The drawing under review shows one solid part. Ordinate dimensions are in mm from its lowest x, y, z. Coordinates: 2 decimals unless noted, no trailing zeros. Write each loop counter-clockwise with the first axis right and the second up, starting at its lowest first coordinate (ties: lowest second). Pieces come first, ordered by that corner, then holes. Notation, with made-up numbers: (-29, 16.25) - (7, 16.25) arc R16 cw to (7, 40.25) - close; hole circle Ø5 at (67, 27). An arc over 180 degrees is marked (long way). Answer as CSV lines item,"result". Start each with the question number.
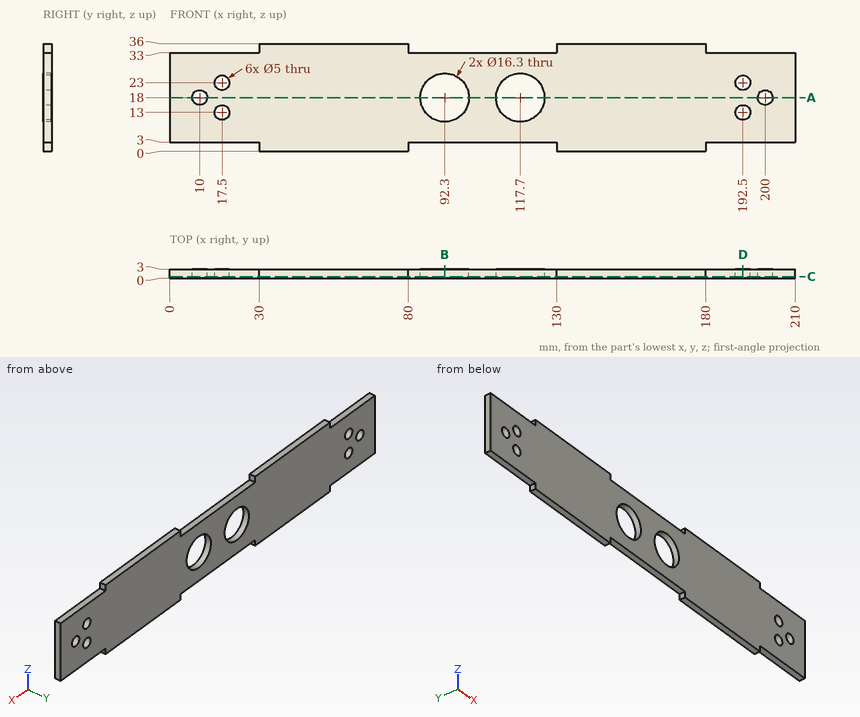
(1) Add section D-D on x = 192.5. Give the boundary of the cut face in (y, z), then the cut area to 3 significant figures.
(2) Add section C-C on y = 0.5. Give the number of separate pieces and of enclosed holes in the cut face, then the cut area to 3 significant figures.
(3) For pin 1 (4 mm diameter, centred on x = 192.5, z = 23, fed in from +Y); pin 2 (1.5 mm diameter, centred on x = 103, y = 1, fed in from -Z); pin 3 (0.9 mm diameter, centred on y = 1, z = 2, fed in from -X), all flat-tipped, find the tip position at first contact; note any pin that passes through.
(4) Add section A-A on z = 18. Give the boundary of the cut face in (x, y), then the cut area to 3 significant figures.
(5) Wall thickness on line 1 (X direction, y = 1.7, z = 18); line 2 (X direction, y = 1.9, z = 23); line 3 (X direction, y = 2.5, z = 2): over which ranges is each line inside the solid? List them lowest first.
(6) Add section B-B on x = 92.3. Give the boundary of the cut face in (y, z).
Reported:
1,outline,"(0, 3) - (3, 3) - (3, 10.5) - (0, 10.5) - close; (0, 15.5) - (3, 15.5) - (3, 20.5) - (0, 20.5) - close; (0, 25.5) - (3, 25.5) - (3, 33) - (0, 33) - close"
1,area,"60.0 mm²"
2,separate pieces,"1"
2,enclosed holes,"8"
2,area,"6,360 mm²"
3,pin 1,"through"
3,pin 2,"z = 3"
3,pin 3,"x = 30"
4,outline,"(0, 0) - (7.5, 0) - (7.5, 3) - (0, 3) - close; (12.5, 0) - (84.15, 0) - (84.15, 3) - (12.5, 3) - close; (100.45, 0) - (109.55, 0) - (109.55, 3) - (100.45, 3) - close; (125.85, 0) - (197.5, 0) - (197.5, 3) - (125.85, 3) - close; (202.5, 0) - (210, 0) - (210, 3) - (202.5, 3) - close"
4,area,"502 mm²"
5,line 1,"0 to 7.5, 12.5 to 84.15, 100.45 to 109.55, 125.85 to 197.5, 202.5 to 210"
5,line 2,"0 to 15, 20 to 85.86, 98.74 to 111.26, 124.14 to 190, 195 to 210"
5,line 3,"30 to 80, 130 to 180"
6,outline,"(0, 3) - (3, 3) - (3, 9.85) - (0, 9.85) - close; (0, 26.15) - (3, 26.15) - (3, 33) - (0, 33) - close"
